Print and shaded views of the part. All mm, measured from the part's lowest x, y and z. Round coordinates to 2 decimals unless told otherwise and drop trailing zeros. Write each loop counter-clockwise with the first axis right and the second up, starting at its lowest first coordinate (ties: lowest second). Pieces come first, ordered by that corner, then holes. Notation, with made-up numbers: (16.5, -16.5) - (23.5, -16.5) arc R10 cw to (23.5, -6.5) - close; hole circle Ø2 at (-35, 41). An arc over 180 degrees is marked (long way). Put each result on its own line as item: value. Start each with the question number.
Item 1: Mould opens along Y. For the marked faces 1, 2 and 3 say: released by +Y, released by -Y, zero draft, split by the parting line, or undercut.
Item 2: Cut at B-B (y = 36.3). Give the cut face in (x, z).
Item 3: Pin check, flat tips, straight feed: pin 1 Ø1.5 at (y, z) = (37.5, 1.5) entering from +X; pin 2 Ø3 at (y, z) = (46, 2.5) entering from -X; pin 3 Ø2.5 at (x, z) = (37, 2.5) entering from +Y. Stop position of each tip, or through.
Item 4: Cut at C-C (z = 0.9). Give the cut face in (x, y), and give its area (3 significant figures).
Item 5: Cut at A-A (x = 36.3). Give the cut face in (y, z).
Item 6: Drill centre lines: line 1 (Y direction, x = 36, z = 3.55); line 2 (X direction, y = 36.5, z = 4.4); line 3 (X direction, y = 33, z = 1.4) (1 decimal). Where is each one in solid material? Low to high. Write a range as from..to.
Item 7: Cut at D-D (y = 68.5). Give the cut face in (x, z) (1 decimal).
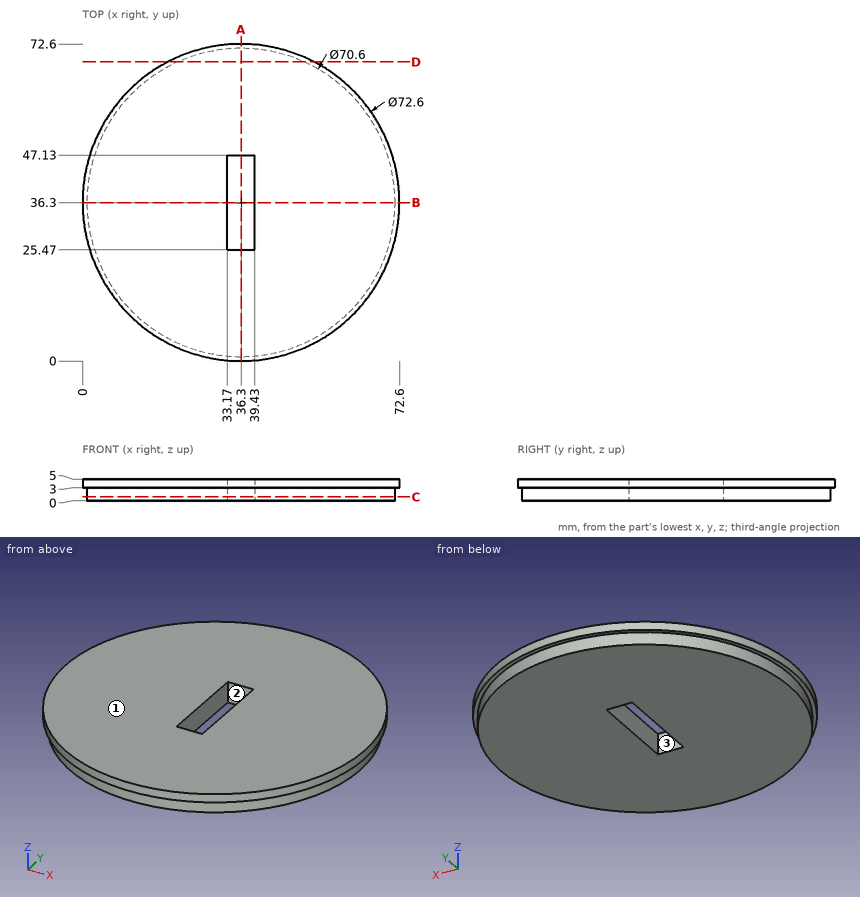
Output values:
1. face 1: zero draft
1. face 2: undercut
1. face 3: undercut
2. outline: (0, 3) - (1, 3) - (1, 0) - (33.17, 0) - (33.17, 5) - (0, 5) - close; (39.43, 0) - (71.6, 0) - (71.6, 3) - (72.6, 3) - (72.6, 5) - (39.43, 5) - close
3. pin 1: x = 71.6
3. pin 2: x = 0.96
3. pin 3: y = 72.6
4. outline: circle Ø70.6 at (36.3, 36.3); hole (33.17, 25.47) - (39.43, 25.47) - (39.43, 47.13) - (33.17, 47.13) - close
4. area: 3,780 mm2
5. outline: (0, 3) - (1, 3) - (1, 0) - (25.47, 0) - (25.47, 5) - (0, 5) - close; (47.13, 0) - (71.6, 0) - (71.6, 3) - (72.6, 3) - (72.6, 5) - (47.13, 5) - close
6. line 1: 0..25.47, 47.13..72.6
6. line 2: 0..33.17, 39.43..72.6
6. line 3: 1.2..33.2, 39.4..71.4
7. outline: (19.5, 3) - (21.8, 3) - (21.8, 0) - (50.8, 0) - (50.8, 3) - (53.1, 3) - (53.1, 5) - (19.5, 5) - close
